from build123d import *

# Parameters (mm, degrees)
EXTRUDE_1_DEPTH     = 3
SKETCH_2_R          = 4
CUT_EXTRUDE_1_DEPTH = 3
CHAMFER_1_SIZE      = 0.1


with BuildPart() as part:
    # 草图1 → 凸台-拉伸1 (new body)
    with BuildSketch(Plane.XY):
        Polygon((0, 7.505553499), (-6.5, 3.75277675), (-6.5, -3.75277675), (0, -7.505553499), (6.5, -3.75277675), (6.5, 3.75277675), align=None)
    extrude(amount=-EXTRUDE_1_DEPTH)

    # 草图2 → 切除-拉伸1 (cut)
    with BuildSketch(Plane.XY):
        Circle(SKETCH_2_R)
    extrude(amount=-CUT_EXTRUDE_1_DEPTH, mode=Mode.SUBTRACT)

    # 倒角1
    chamfer_1_edges = [part.edges().sort_by_distance(p)[0] for p in [
        (-4, 0, -3),
        (-4, 0, 0),
    ]]
    chamfer(chamfer_1_edges, length=CHAMFER_1_SIZE)


solid = part.part
Here's how the part is built. I have some questions about the finished solid (model axes, mm). Coordinates: 2 decimals unless noted, no trailing zeros. Write each loop counter-clockwise with the first axis right and the second up, starting at its lowest first coordinate (ties: lowest second). Pieces come first, ordered by that corner, then holes.
1) If I drill on line 1 (Y direction, x = 3, z = -1.1); line 2 (X direction, y = -0.75, z = -0.65); line 3 (X direction, y = 2.5, z = -1.15), over which ranges is the centre line in solid material (lowest first)?
Filled in:
line 1: y = -5.77 to -2.65, 2.65 to 5.77
line 2: x = -6.5 to -3.93, 3.93 to 6.5
line 3: x = -6.5 to -3.12, 3.12 to 6.5
2) If we section it at A-A (y = 0): List the corners of the cut face in (x, z) for me.
Filled in:
outline: (-6.5, -3) - (-4.1, -3) - (-4, -2.9) - (-4, -0.1) - (-4.1, 0) - (-6.5, 0) - close; (4, -2.9) - (4.1, -3) - (6.5, -3) - (6.5, 0) - (4.1, 0) - (4, -0.1) - close
3) Thinking about a two-plate mould opening in Y: for faces 1 (the face through (-0.867, -3.905, -1.48)), 2 (the face through (-3.3, -5.6, -1.5)), 3 (the face through (2.8, -3.2, 0)), which applies, +Y half, -Y half, draft (parallel to the pull), parting line (faces both ways), or undercut?
Filled in:
face 1: undercut
face 2: -Y half
face 3: draft
4) If we section it at C-C (y = 5.5): List the corners of the cut face in (x, z) for me.
Filled in:
outline: (-3.47, -3) - (3.47, -3) - (3.47, 0) - (-3.47, 0) - close
5) I'm going to push flat-ended pins straight in: pin 1 (1 mm diameter, centred on x = 1.5, z = -2.5, fed in from -Y); pin 2 (1.5 mm diameter, centred on x = -4.5, z = -1.5, fed in from -Y). Where does each tip first touch, or does it pass through?
Filled in:
pin 1: stops at y = -6.93
pin 2: stops at y = -5.34
6) If we section it at B-B (z = -0.95): List the corners of the cut face in (x, y) for me.
Filled in:
outline: (-6.5, -3.75) - (0, -7.51) - (6.5, -3.75) - (6.5, 3.75) - (0, 7.51) - (-6.5, 3.75) - close; hole circle Ø8 at (0, 0)
